Input: part model. Units: mm. Frame: model coordinates. A direction names the side the tool comes from. Coordinates: 2 decimals unless noted, no trailing zeros. Order: outer loops, then holes, each group sorted by start corner. A loop starts at its lowest first (then second) coordinate and runs counter-clockwise, first axis right, second up. Notation, with made-up numbers: (72.25, -30.75) -> (119.25, -30.75) arc R26 cw to (119.25, 6.25) -> close; hole circle Ø4 at (5.5, 8.25). An arc over 180 degrees is marked (long way). Answer as CSV lines item,"result".
from build123d import *

# Parameters (mm, degrees)
SKETCH_2_W          = 5.8
SKETCH_2_H          = 0.8
CUT_EXTRUDE_1_DEPTH = 1.5
FILLET_1_R          = 0.2


with BuildPart() as part:
    # 草图1 → 旋转1 (revolve)
    with BuildSketch(Plane.XY):
        with BuildLine():
            Line((2.4, 2.9), (2.4, 1.5))
            Line((2.4, 1.5), (10.4, 1.5))
            Line((10.4, 1.5), (24.4, 1.5))
            Line((24.4, 1.5), (24.4, 0))
            Line((24.4, 0), (0, 0))
            ThreePointArc((0, 0), (0.677815098, 1.882153022), (2.4, 2.9))
        make_face()
    revolve(axis=Axis((0, 0, 0), (1, 0, 0)))

    # 草图2 → 切除-拉伸1 (cut)
    with BuildSketch(Plane(origin=(0, 0, 0), x_dir=(0, 0, -1), z_dir=(1, 0, 0))):
        Rectangle(SKETCH_2_W, SKETCH_2_H)
    extrude(amount=CUT_EXTRUDE_1_DEPTH, mode=Mode.SUBTRACT)

    # 圆角1
    fillet_1_edges = [part.edges().sort_by_distance(p)[0] for p in [
        (2.4, -1.5, 0),
    ]]
    fillet(fillet_1_edges, radius=FILLET_1_R)


solid = part.part
1. Reachability of faces 4 (the face through (2.4, 0, -2)), 5 (the face through (1, -0.4, 0)) from +Z, -Z, +X, -X, +Y, -Y: full face, straight path, thin tool, end or side. Return the list, or none.
Findings:
face 4,"+X"
face 5,"+Z, -Z, -X"
2. Mould query, pull axis Y, two halves, no side actions, for faces 1 (the face through (24.4, 0, 0)), 2 (the face through (13.65, -1.5, 0.07)), 3 (the face through (1, 0.4, 0)). Classes: released by +Y, released by -Y, zero draft, split by the parting line, or undercut.
Findings:
face 1,"zero draft"
face 2,"split by the parting line"
face 3,"undercut"
3. Ray query, line 1 along X through (y, z) = (0.35, -2.4); line 2 along X through (y, z) = (-0.15, -1.45); line 3 along Y through (x, z) = (5.75, -1.15). Return the intervals inside material, ascending.
Findings:
line 1,"x = 1.5 to 2.4"
line 2,"x = 1.5 to 24.4"
line 3,"y = -0.96 to 0.96"
4. Cut plane B-B (y = 0). Return the cut outline in (x, z), plus the area to 3 significant figures.
Findings:
outline,"(1.5, -2.57) arc R2.95 ccw to (2.4, -2.9) -> (2.4, -1.7) arc R0.2 cw to (2.6, -1.5) -> (24.4, -1.5) -> (24.4, 1.5) -> (2.6, 1.5) arc R0.2 cw to (2.4, 1.7) -> (2.4, 2.9) arc R2.95 ccw to (1.5, 2.57) -> close"
area,"71.0 mm2"
5. Contact query for flat-ended pins moving along their axis: pin 1 (0.7 mm diameter, centred on x = 1, z = 1, fed in from -Y); pin 2 (1.6 mm diameter, centred on x = 0.5, z = 0, fed in from +Y); pin 3 (1.5 mm diameter, centred on y = -1.5, z = 2.5, fed in from +X). Output: stop coordinate, or through.
Findings:
pin 1,"stops at y = -2.31"
pin 2,"stops at y = 2.45"
pin 3,"stops at x = 2.4"
6. Cut plane A-A (z = 0). Return the cut outline in (x, y), plus the area to 3 significant figures.
Findings:
outline,"(0.03, -0.4) arc R2.95 ccw to (2.4, -2.9) -> (2.4, -1.7) arc R0.2 cw to (2.6, -1.5) -> (24.4, -1.5) -> (24.4, 1.5) -> (2.6, 1.5) arc R0.2 cw to (2.4, 1.7) -> (2.4, 2.9) arc R2.95 ccw to (0.03, 0.4) -> (1.5, 0.4) -> (1.5, -0.4) -> close"
area,"75.3 mm2"
7. Cut plane D-D (y = -2.35). Return the cut outline in (x, z).
Findings:
outline,"(2.4, -1.7) -> (2.4, 1.7) arc R1.79 ccw to start"
8. Cut plane C-C (x = 11.25). Return the cut outline in (y, z).
Findings:
outline,"circle Ø3 at (0, 0)"
